Read the model definition and answer for the solid it produces. Units are mm, in the model's axes. Face numbers are marked on the shaded views. A direction names the side the tool comes from. Coordinates: 2 decimals unless noted, no trailing zeros. Loops run counter-clockwise (first coordinate to the right, second up) from the corner with the lowest first, then second, coordinate; pieces in that order, holes last. Notation, with made-up numbers: (1.25, 14) - (54.25, 14) arc R24 ccw to (54.25, 48) - close; hole circle Ø1 at (32.25, 13.25). An arc over 180 degrees is marked (long way). One line per item, written item: value. Start each with the question number.
from build123d import *

# Parameters (mm, degrees)
F0_R     = 44.4983776942
F1_DEPTH = 110.49
F2_R     = 14.5195610464
F3_DEPTH = 202.946
F4_SIZE  = 5.08
F5_R     = 5.08
F6_W     = 128.777243197
F6_H     = 130.6803599
F7_DEPTH = 77.47


with BuildPart() as f1:
    # F0 (on Front) → F1 (new body)
    with BuildSketch(Plane.XZ):
        Circle(F0_R)
    extrude(amount=F1_DEPTH)

    # F2 (on Front) → F3 (cut)
    with BuildSketch(Plane.XZ):
        with Locations((1.9654189236, 0)):
            Circle(F2_R)
    extrude(amount=F3_DEPTH, mode=Mode.SUBTRACT)

    # F4
    f4_edges = [f1.edges().sort_by_distance(p)[0] for p in [
        (-12.554142, -110.49, 0),
        (-12.554142, 0, 0),
        (-44.498378, -110.49, 0),
        (-44.498378, 0, 0),
    ]]
    chamfer(f4_edges, length=F4_SIZE)

    # F5
    f5_edges = [f1.edges().sort_by_distance(p)[0] for p in [
        (-44.498378, -105.41, 0),
        (-39.418378, -110.49, 0),
        (-44.498378, -5.08, 0),
        (-39.418378, 0, 0),
        (-12.554142, -105.41, 0),
        (-17.634142, -110.49, 0),
        (19.02498, -2.54, 0),
        (-17.634142, 0, 0),
        (-12.554142, -5.08, 0),
    ]]
    fillet(f5_edges, radius=F5_R)

    # F6 (on Front) → F7 (join)
    with BuildSketch(Plane.XZ):
        with Locations((-1.7445199192, -5.1542632282)):
            Rectangle(F6_W, F6_H)
    extrude(amount=-F7_DEPTH)


solid = f1.part
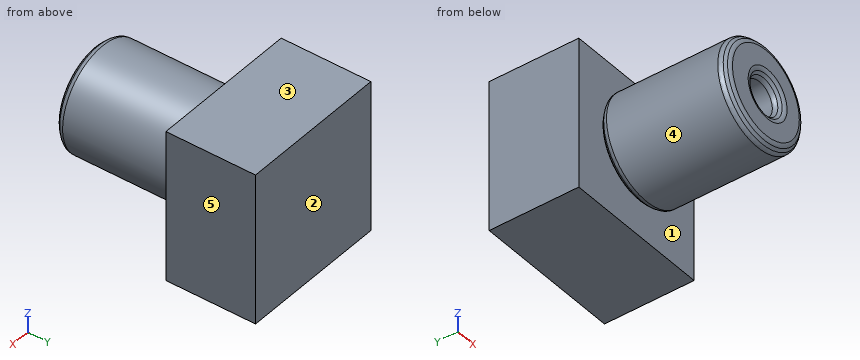
1) Section A-A, the plane y = -98 is taken. Determine the outline of the cut face in (x, z), and give its area (3 significant figures).
2) Flat-ended cylindrical pins translate along their axes: P1, Ø2, axis at y = -6, z = -34, coming from the -X side; P2, Ø2, axis at x = 6.5, y = -54.5, coming from the -Z side; P3, Ø10, axis at x = -33, z = -46, coming from the -Y side. Find the tip coordinate at first contact, or state that the pin passes through.
3) Determine the mould class of the marked faces 1, 2 and 3 for opening direction Y: released by +Y, released by -Y, zero draft, split by the parting line, or undercut.
4) Section C-C, the plane x = 48 is taken. Determine the outline of the cut face in (y, z), and give its area (3 significant figures).
5) For the marked faces 4 and 5, determine the directions among +Z, -Z, +X, -X, +Y, -Y from which every point of the face is accessible in a straight line to the end or side of a thin tool.
6) Section B-B, the plane z = -54.5 is taken. Determine the outline of the cut face in (x, y), and give its area (3 significant figures).
7) Straight lines are drawn through the part: L1, parallel to X at y = -69, z = 0; L2, parallel to Y at x = 26, z = -40; L3, parallel to Y at x = -1, z = 42. For each, find the intervals that lie inside material, in ascending order.
Answer below:
1. outline: circle Ø89 at (0, 0); hole circle Ø29.04 at (1.97, 0)
1. area: 5,560 mm2
2. P1: x = -29.69
2. P2: z = -44.16
2. P3: y = 0
3. face 1: undercut
3. face 2: released by +Y
3. face 3: zero draft
4. outline: (0, -70.49) - (77.47, -70.49) - (77.47, 60.19) - (0, 60.19) - close
4. area: 10,100 mm2
5. face 4: -Y
5. face 5: +Z, -Z, +X, +Y, -Y
6. outline: (-66.13, 0) - (62.64, 0) - (62.64, 77.47) - (-66.13, 77.47) - close
6. area: 9,980 mm2
7. L1: -44.5 to -12.55, 16.48 to 44.5
7. L2: 0 to 77.47
7. L3: -107.9 to -2.59, 0 to 77.47
